Can you work these out from the model? Positions are in its coordinate system, mm. Face numbers are marked on the shaded views. A direction names the side the tool comes from. Give positions to 0.01 mm unless a question says otherwise; leave off trailing zeros. Order: outer loops, then holes, each group sorted by start corner. A loop starts at its lowest first (then second) coordinate and runs counter-clockwise, first axis right, second up. Notation, with made-up numbers: M 68,-30.75 L 92,-30.75 A30 ccw 92,2.25 Z; hole C 85.25,-14.75 d7. An arc over 180 degrees is marked long. One line per question, with ' | ' between items. Start each with the question number.
1) Please list where these lines run through material, in increasing order: line 1 along Z through (x, y) = (-18, 5.5); line 2 along X through (y, z) = (6.5, 0.75); line 3 along Z through (x, y) = (19, 5). Write a range as [from, to].
2) If we section it at D-D, the plane x = 9.5: Please give me the cut outline in (y, z), plus the area to 3 significant figures.
3) If we section it at B-B, the plane x = 19: Please give me the cut outline in (y, z).
4) If we section it at A-A, the plane z = 0: Please give me the cut outline in (x, y).
5) If we section it at C-C, the plane y = 3.75: Please give me the cut outline in (x, z).
6) I'm going to push flat-ended pins straight in: pin 1 Ø1 at (x, y) = (17, 6.5) entering from -Z; pin 2 Ø6.5 at (x, z) = (-18, 0) entering from -Y. Where does each tip first touch, or does it pass through?
7) Thinking about a two-plate mould opening in Z: for the marked faces 1, 2, 3 and 4, which applies, +Z half, -Z half, draft (parallel to the pull), parting line (faces both ways), or undercut?
8) For the marked faces 5 and 6, which set-ups out of +Z, -Z, +X, -X, +Y, -Y let a thin tool reach every point of the face, with its end or its side?
```python
from build123d import *

# Parameters (mm, degrees)
SKETCH2_W           = 50
SKETCH2_H           = 14
BOSS_EXTRUDE1_DEPTH = 8
SKETCH3_R           = 2.5
CUT_EXTRUDE2_DEPTH  = 9
FILLET5_R           = 2


with BuildPart() as part:
    # Sketch2 → Boss-Extrude1 (new body)
    with BuildSketch(Plane(origin=(0, 0, 0), x_dir=(1, 0, 0), z_dir=(0, 1, 0))):
        Rectangle(SKETCH2_W, SKETCH2_H)
    extrude(amount=BOSS_EXTRUDE1_DEPTH)

    # Sketch3 → Cut-Extrude2 (cut, symmetric)
    with BuildSketch(Plane(origin=(0, 8, 0), x_dir=(1, 0, 0), z_dir=(0, 1, 0))):
        with Locations((19, 0)):
            Circle(SKETCH3_R)
        with BuildLine():
            Line((-21.307189139, 2.25), (-21.307189139, -2.25))
            ThreePointArc((-21.307189139, -2.25), (-14, 0), (-21.307189139, 2.25))
        make_face()
    extrude(amount=CUT_EXTRUDE2_DEPTH, both=True, mode=Mode.SUBTRACT)

    # Fillet5
    fillet5_edges = [part.edges().sort_by_distance(p)[0] for p in [
        (-25, 8, 0),
        (0, 8, 7),
        (25, 8, 0),
        (0, 0, 7),
        (-25, 0, 0),
        (0, 0, -7),
        (25, 0, 0),
        (0, 8, -7),
    ]]
    fillet(fillet5_edges, radius=FILLET5_R)


solid = part.part
```
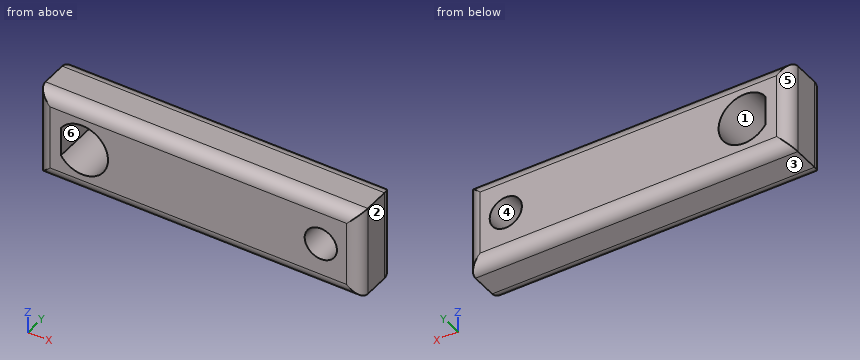
Results found:
1) line 1: z = [-7, -4], [4, 7] | line 2: x = [-24.94, -21.31], [-14.07, 16.62], [21.38, 24.94] | line 3: z = [-7, -2.5], [2.5, 7]
2) outline: M 0,-5 A2 ccw 2,-7 L 6,-7 A2 ccw 8,-5 L 8,5 A2 ccw 6,7 L 2,7 A2 ccw 0,5 Z | area: 109 mm²
3) outline: M 0,-5 A2 ccw 2,-7 L 6,-7 A2 ccw 8,-5 L 8,-2.5 L 0,-2.5 Z; M 0,2.5 L 8,2.5 L 8,5 A2 ccw 6,7 L 2,7 A2 ccw 0,5 Z
4) outline: M -25,2 A2 ccw -23,0 L -21.31,0 L -21.31,8 L -23,8 A2 ccw -25,6 Z; M -14,0 L 16.5,0 L 16.5,8 L -14,8 Z; M 21.5,0 L 23,0 A2 ccw 25,2 L 25,6 A2 ccw 23,8 L 21.5,8 Z
5) outline: M -25,-7 L 25,-7 L 25,7 L -25,7 Z; hole M -21.31,-2.25 A4 ccw long -21.31,2.25 Z; hole C 19,0 d5
6) pin 1: stops at z = -7 | pin 2: passes through
7) face 1: undercut | face 2: draft | face 3: -Z half | face 4: undercut
8) face 5: +Z, -Z, -X, +Y | face 6: +Y, -Y
